from build123d import *

# Parameters (mm, degrees)
CROQUIS1_R              = 25
SALIENTE_EXTRUIR1_DEPTH = 30


with BuildPart() as part:
    # Croquis1 → Saliente-Extruir1 (new body)
    with BuildSketch(Plane(origin=(0, 0, 0), x_dir=(1, 0, 0), z_dir=(0, 1, 0))):
        with BuildLine():
            ThreePointArc((-4.993746089, 49.75), (-35.355339059, 35.355339059), (-49.75, 4.993746089))
            ThreePointArc((-49.75, 4.993746089), (-55, 0), (-49.75, -4.993746089))
            ThreePointArc((-49.75, -4.993746089), (-35.355339059, -35.355339059), (-4.993746089, -49.75))
            ThreePointArc((-4.993746089, -49.75), (0, -55), (4.993746089, -49.75))
            ThreePointArc((4.993746089, -49.75), (35.355339059, -35.355339059), (49.75, -4.993746089))
            ThreePointArc((49.75, -4.993746089), (55, 0), (49.75, 4.993746089))
            ThreePointArc((49.75, 4.993746089), (35.355339059, 35.355339059), (4.993746089, 49.75))
            ThreePointArc((4.993746089, 49.75), (0, 55), (-4.993746089, 49.75))
        make_face()
        with Locations(Location((0, 0, 0), (0, 0, 270))):  # turned: the seam where the file's is
            Circle(CROQUIS1_R, mode=Mode.SUBTRACT)
    extrude(amount=SALIENTE_EXTRUIR1_DEPTH)


solid = part.part
Could you check a few things on this model? Use its own coordinates, in mm. Give positions to 0.01 mm unless a question says otherwise; leave off trailing zeros. Order: outer loops, then holes, each group sorted by start corner. A loop starts at its lowest first (then second) coordinate and runs counter-clockwise, first axis right, second up.
1. Suppose I cut it at C-C (z = -23). Write out the boundary of the cut face in (x, y), plus the area to 3 significant figures.
Answers below:
outline: (-44.4, 0) - (-9.8, 0) - (-9.8, 30) - (-44.4, 30) - close; (9.8, 0) - (44.4, 0) - (44.4, 30) - (9.8, 30) - close
area: 2,080 mm2
2. For pin 1 (2 mm diameter, centred on x = -2, z = 41.5, fed in from -Y); pin 2 (2 mm diameter, centred on x = -20, y = 9.5, fed in from +Z); pin 3 (10 mm diameter, centred on y = 19, z = -37.5, fed in from -X); pin 4 (1.5 mm diameter, centred on x = 14.5, y = 19.5, fed in from -Z), each with a flat end and sliding along its axis, tell me the tip position at first contact or that it passes through.
Answers below:
pin 1: stops at y = 0
pin 2: stops at z = 46.25
pin 3: stops at x = -38
pin 4: stops at z = -48.07
3. Suppose I cut it at B-B (x = 0). Write out the boundary of the cut face in (y, z).
Answers below:
outline: (0, -55) - (30, -55) - (30, -25) - (0, -25) - close; (0, 25) - (30, 25) - (30, 55) - (0, 55) - close
4. I need wall thicknesses on L1, parallel to X at y = 12.25, z = 0; L2, parallel to X at y = 11.75, z = 15; L3, parallel to Z at x = -13.5, y = 9.5. Which ranges of each line are inside material? Lowest first, please.
Answers below:
L1: x = -55 to -25, 25 to 55
L2: x = -47.7 to -20, 20 to 47.7
L3: z = -48.14 to -21.04, 21.04 to 48.14
5. Suppose I cut it at D-D (z = 35). Write out the boundary of the cut face in (x, y), plus the area to 3 significant figures.
Answers below:
outline: (-35.71, 0) - (35.71, 0) - (35.71, 30) - (-35.71, 30) - close
area: 2,140 mm2
6. Thinking about a two-plate mould opening in X: for faces 1 (the flat face through (24, 0, 11)), 2 (the cylindrical face through (7.509, 14.79, 23.846)), 3 (the cylindrical face through (35.693, 14.79, -35.014)), which applies, +X half, -X half, draft (parallel to the pull), parting line (faces both ways), or undercut?
Answers below:
face 1: draft
face 2: undercut
face 3: +X half
7. Suppose I cut it at A-A (y = 20.5). Write out the boundary of the cut face in (x, z), plus the area to 3 significant figures.
Answers below:
outline: (-49.75, -4.99) arc R50 ccw to (-4.99, -49.75) arc R5 ccw (long way) to (4.99, -49.75) arc R50 ccw to (49.75, -4.99) arc R5 ccw (long way) to (49.75, 4.99) arc R50 ccw to (4.99, 49.75) arc R5 ccw (long way) to (-4.99, 49.75) arc R50 ccw to (-49.75, 4.99) arc R5 ccw (long way) to start; hole circle Ø50 at (0, 0)
area: 6,050 mm2
